from build123d import *

# Parameters (mm, degrees)
BASEPLATE_W                      = 200
BASEPLATE_H                      = 200
BOSS_EXTRUDE1_DEPTH              = 9.5
FILLET1_R                        = 9.5
F_1_4_INCH_BOLT_HOLE_D           = 6.35
F_1_4_INCH_BOLT_HOLE_CSINK_D     = 7.62
F_1_4_INCH_BOLT_HOLE_CSINK_ANGLE = 90
F_5_32_DOWEL_HOLE_D              = 3.96875
F_5_32_DOWEL_HOLE_DEPTH          = 6
F_5_32_DOWEL_HOLE_CSINK_D        = 5.23875
F_5_32_DOWEL_HOLE_CSINK_ANGLE    = 100
F_5_32_DOWEL_HOLE_TIP            = 1.192332791


with BuildPart() as part:
    # Baseplate → Boss-Extrude1 (new body)
    with BuildSketch(Plane.XY):
        Rectangle(BASEPLATE_W, BASEPLATE_H)
    extrude(amount=BOSS_EXTRUDE1_DEPTH)

    # Fillet1
    fillet1_edges = [part.edges().sort_by_distance(p)[0] for p in [
        (100, -100, 4.75),
        (-100, -100, 4.75),
        (-100, 100, 4.75),
        (100, 100, 4.75),
    ]]
    fillet(fillet1_edges, radius=FILLET1_R)

    # 1/4 Inch Bolt Hole (through all)
    with Locations(Plane(origin=(0, 0, 0), x_dir=(-1, 0, 0), z_dir=(0, 0, -1))):
        with Locations((0, 0)):
            CounterSinkHole(F_1_4_INCH_BOLT_HOLE_D / 2, F_1_4_INCH_BOLT_HOLE_CSINK_D / 2, counter_sink_angle=F_1_4_INCH_BOLT_HOLE_CSINK_ANGLE)

    # 5/32 Dowel Hole
    with Locations(Plane(origin=(0, 0, 0), x_dir=(-1, 0, 0), z_dir=(0, 0, -1))):
        with Locations((-44.5, 0), (44.45, 0)):
            CounterSinkHole(F_5_32_DOWEL_HOLE_D / 2, F_5_32_DOWEL_HOLE_CSINK_D / 2, depth=F_5_32_DOWEL_HOLE_DEPTH, counter_sink_angle=F_5_32_DOWEL_HOLE_CSINK_ANGLE)
            with Locations((0, 0, -(F_5_32_DOWEL_HOLE_DEPTH + F_5_32_DOWEL_HOLE_TIP / 2))):  # 118° drill point
                Cone(0, F_5_32_DOWEL_HOLE_D / 2, F_5_32_DOWEL_HOLE_TIP, mode=Mode.SUBTRACT)


solid = part.part
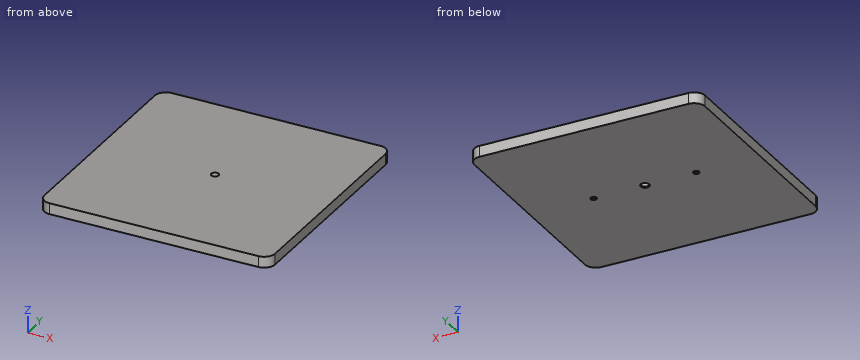
Source: CAD feature listing. Evaluate the final solid. Frame: model axes, mm. Round coordinates to 2 decimals unless told otherwise and drop trailing zeros. Order: outer loops, then holes, each group sorted by start corner. A loop starts at its lowest first (then second) coordinate and runs counter-clockwise, first axis right, second up. Notation, with made-up numbers: (3.5, 50.25) - (19.5, 50.25) arc R20 cw to (19.5, 61.25) - close; hole circle Ø10 at (-19, -17). An arc over 180 degrees is marked (long way). Use a Markdown table: item, result. Add a question column.
1. Section query A-A (x = 0). Return the cut outline in (y, z) (3 decimals), then the cut area to 3 significant figures.
2. First-contact query: pin 1 (2 mm diameter, centred on x = -36, y = 48.5, fed in from -Z); pin 2 (5 mm diameter, centred on x = 44.5, y = 0, fed in from -Z); pin 3 (5 mm diameter, centred on x = 0, y = 0, fed in from -Z). Flat tips, straight axial feed; report the tip coordinate or a pass-through.
3. Line query: probe 1 along X at (y, z) = (0, 4.9) (3 decimals); probe 2 along Y at (x, z) = (-44.45, 2); probe 3 along Y at (x, z) = (0, 7.5) (3 decimals). Output: solid intervals per line, ascending.
Derived:
| question | item | result |
|---|---|---|
| 1 | outline | (-100, 0) - (-3.81, 0) - (-3.175, 0.635) - (-3.175, 9.5) - (-100, 9.5) - close; (3.175, 0.635) - (3.81, 0) - (100, 0) - (100, 9.5) - (3.175, 9.5) - close |
| 1 | area | 1,840 mm2 |
| 2 | pin 1 | z = 0 |
| 2 | pin 2 | z = 0.1 |
| 2 | pin 3 | through |
| 3 | probe 1 | -100 to -46.434, -42.466 to -3.175, 3.175 to 42.516, 46.484 to 100 |
| 3 | probe 2 | -100 to -1.98, 1.98 to 100 |
| 3 | probe 3 | -100 to -3.175, 3.175 to 100 |
